Study the drawing (mm; zero at the part's minimum x, y, z) and answer. A direction names the side the tool comes from. Coordinates: 2 decimals unless noted, no trailing zeros. Write each loop counter-clockwise with the first axis right and the second up, starting at its lowest first coordinate (ties: lowest second). Pieces come first, ordered by that corner, then holes. Notation, with made-up numbers: (-8, -32.5) -> (11, -32.5) arc R9 cw to (11, -20.5) -> close; hole circle Ø10 at (63, 43.5). An arc over 180 degrees is marked (long way). Write item = value, one per line. Start each with the question number.
1) Section D-D (y = 19.25) is taken. Determine the outline of the cut face in (x, z) (1 decimal).
2) Find the intervals of material crossed by line 1 along X through (y, z) = (6.5, 2); line 2 along X through (y, z) = (14.5, 6.25); line 3 along Y through (x, z) = (9, 10.75), in increasing order. Write a range as from..to.
3) Section B-B (y = 15.25) is taken. Determine the outline of the cut face in (x, z).
4) Section A-A (z = 9.25) is taken. Determine the outline of the cut face in (x, y) (1 decimal).
5) Section C-C (x = 16.5) is taken. Determine the outline of the cut face in (y, z) (1 decimal).
6) A tool of negligible diameter and unlimited length cuts with its end or side. For the marked faces 1 and 2, from which of +Z, -Z, +X, -X, +Y, -Y can it reach the whole face along a straight path? Write none if from no direction.
7) Flat-ended cylindrical pins translate along their axes: pin 1 Ø6 at (x, y) = (19, 16.5) entering from +Z; pin 2 Ø1 at (y, z) = (18.5, 8) entering from -X; pin 3 Ø3 at (x, z) = (11, 4.5) entering from -Y; pin 4 Ø5 at (x, z) = (22.5, 3) entering from -Y. Find the tip coordinate at first contact, or state that the pin passes through.
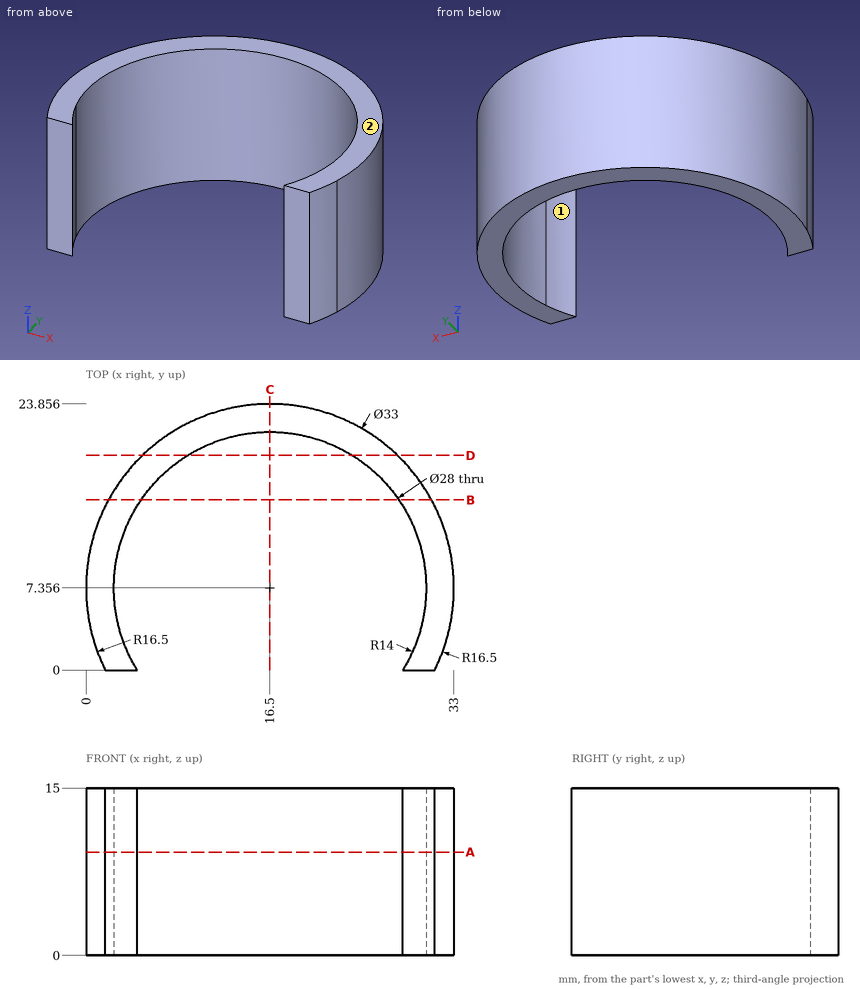
Answer key:
q1.outline = (5.1, 0) -> (9.1, 0) -> (9.1, 15) -> (5.1, 15) -> close; (23.9, 0) -> (27.9, 0) -> (27.9, 15) -> (23.9, 15) -> close
q2.line_1 = 0.02..2.53, 30.47..32.98
q2.line_2 = 1.63..4.46, 28.54..31.37
q2.line_3 = 19.18..22.05
q3.outline = (2.01, 0) -> (4.94, 0) -> (4.94, 15) -> (2.01, 15) -> close; (28.06, 0) -> (30.99, 0) -> (30.99, 15) -> (28.06, 15) -> close
q4.outline = (0.5, 3.4) arc R16.5 ccw to (1.7, 0) -> (4.6, 0) arc R14 cw to (3.1, 3.4) arc R14 cw (long way) to (29.9, 3.4) arc R14 cw to (28.4, 0) -> (31.3, 0) arc R16.5 ccw to (32.5, 3.4) arc R16.5 ccw (long way) to start
q5.outline = (21.4, 0) -> (23.9, 0) -> (23.9, 15) -> (21.4, 15) -> close
q6.face_1 = +Z, -Z
q6.face_2 = +Z, +X, -X, +Y, -Y
q7.pin_1 = through
q7.pin_2 = 3.89
q7.pin_3 = 19.48
q7.pin_4 = 18.48
